Here's how the part is built. I have some questions about the finished solid (model axes, mm). Give positions to 0.01 mm unless a question says otherwise; leave off trailing zeros. Loops run counter-clockwise (first coordinate to the right, second up) from the corner with the lowest first, then second, coordinate; pieces in that order, holes last.
Q1. We'd pull the mould along X, two halves only. Please class faces 1 (the face through (27.9, 0.49, -0.09)), 2 (the face through (-1, 4, 29)), 3 (the face through (-11.548, 0.493, 23.581)), 4 (the face through (30.22, 1.97, 39.34)): +X half, -X half, draft (parallel to the pull), parting line (faces both ways), or undercut.
Q2. Will these pins go through, and if not, where does the flat tip stop? P1, Ø6.5, axis at x = 30, z = 0, coming from the +Y side; P2, Ø5.5, axis at x = -10, z = 55, coming from the +Y side; P3, Ø1.5, axis at y = 3, z = 26.5, coming from the +X side.
Q3. If we section it at D-D (x = 10): Please give me the cut outline in (y, z).
Q4. If we section it at A-A (x = 0): Please give me the cut outline in (y, z), plus the area to 3 significant figures.
Q5. If we section it at C-C (y = 2): Please give me the cut outline in (x, z).
Q6. I need wall thicknesses on line 1 (X direction, y = 0.45, z = 0); line 2 (Z direction, x = 9, y = 2.8); line 3 (Z direction, x = 10, y = 0.4). Which ranges of each line are inside material? Lowest first, please.
Q7. If we section it at B-B (z = 55): Please give me the cut outline in (x, y).
from build123d import *

# Parameters (mm, degrees)
SKETCH1_W           = 40
SKETCH1_H           = 60
SKETCH1_R           = 2.1
SKETCH1_W_2         = 80
SKETCH1_H_2         = 20
BOSS_EXTRUDE1_DEPTH = 4
CHAMFER1_SIZE       = 3
FILLET1_R           = 4


with BuildPart() as part:
    # Sketch1 → Boss-Extrude1 (new body)
    with BuildSketch(Plane(origin=(0, 0, 0), x_dir=(1, 0, 0), z_dir=(0, 1, 0))):
        with Locations((0, -40)):
            Rectangle(SKETCH1_W, SKETCH1_H)
        with Locations((-10, -55)):
            Circle(SKETCH1_R, mode=Mode.SUBTRACT)
        with Locations((10, -55)):
            Circle(SKETCH1_R, mode=Mode.SUBTRACT)
        with Locations((-10, -25)):
            Circle(SKETCH1_R, mode=Mode.SUBTRACT)
        with Locations((10, -25)):
            Circle(SKETCH1_R, mode=Mode.SUBTRACT)
        Polygon((-20, -10), (-40, -10), (-20, -70), align=None)
        Polygon((40, -10), (20, -10), (20, -70), align=None)
        Rectangle(SKETCH1_W_2, SKETCH1_H_2)
        Circle(SKETCH1_R, mode=Mode.SUBTRACT)
        with Locations((30, 0)):
            Circle(SKETCH1_R, mode=Mode.SUBTRACT)
        with Locations((-30, 0)):
            Circle(SKETCH1_R, mode=Mode.SUBTRACT)
    extrude(amount=BOSS_EXTRUDE1_DEPTH)

    # Chamfer1
    chamfer1_edges = [part.edges().sort_by_distance(p)[0] for p in [
        (-12.1, 4, 55),
        (7.9, 4, 55),
        (7.9, 4, 25),
        (-12.1, 4, 25),
        (-2.1, 4, 0),
        (27.9, 4, 0),
        (-32.1, 4, 0),
    ]]
    chamfer(chamfer1_edges, length=CHAMFER1_SIZE)

    # Fillet1
    fillet1_edges = [part.edges().sort_by_distance(p)[0] for p in [
        (20, 2, 70),
        (-20, 2, 70),
        (-40, 2, 10),
        (-40, 2, -10),
        (40, 2, -10),
        (40, 2, 10),
    ]]
    fillet(fillet1_edges, radius=FILLET1_R)


solid = part.part
Check sheet entries:
1. face 1: undercut
1. face 2: draft
1. face 3: undercut
1. face 4: +X half
2. P1: stops at y = 2.15
2. P2: stops at y = 1.65
2. P3: stops at x = 34.75
3. outline: (0, -10) - (4, -10) - (4, 19.9) - (1, 22.9) - (0, 22.9) - close; (0, 27.1) - (1, 27.1) - (4, 30.1) - (4, 49.9) - (1, 52.9) - (0, 52.9) - close; (0, 57.1) - (1, 57.1) - (4, 60.1) - (4, 70) - (0, 70) - close
4. outline: (0, -10) - (4, -10) - (4, -5.1) - (1, -2.1) - (0, -2.1) - close; (0, 2.1) - (1, 2.1) - (4, 5.1) - (4, 70) - (0, 70) - close
4. area: 294 mm2
5. outline: (-40, -6) arc R4 ccw to (-36, -10) - (36, -10) arc R4 ccw to (40, -6) - (40, 9.35) arc R4 ccw to (39.79, 10.62) - (20.91, 67.26) arc R4 ccw to (17.12, 70) - (-17.12, 70) arc R4 ccw to (-20.91, 67.26) - (-39.79, 10.62) arc R4 ccw to (-40, 9.35) - close; hole circle Ø6.2 at (-30, 0); hole circle Ø6.2 at (-10, 25); hole circle Ø6.2 at (-10, 55); hole circle Ø6.2 at (0, 0); hole circle Ø6.2 at (10, 25); hole circle Ø6.2 at (10, 55); hole circle Ø6.2 at (30, 0)
6. line 1: x = -40 to -32.1, -27.9 to -2.1, 2.1 to 27.9, 32.1 to 40
6. line 2: z = -10 to 21.23, 28.77 to 51.23, 58.77 to 70
6. line 3: z = -10 to 22.9, 27.1 to 52.9, 57.1 to 70
7. outline: (-25, 0) - (-12.1, 0) - (-12.1, 1) - (-15.1, 4) - (-25, 4) - close; (-7.9, 0) - (7.9, 0) - (7.9, 1) - (4.9, 4) - (-4.9, 4) - (-7.9, 1) - close; (12.1, 0) - (25, 0) - (25, 4) - (15.1, 4) - (12.1, 1) - close
